from build123d import *

# Parameters (mm, degrees)
BOSS_EXTRUDE6_DEPTH  = 1.27
SKETCH3_R            = 2.54
SKETCH3_R_2          = 1.27
BOSS_EXTRUDE8_DEPTH  = 0.635
BOSS_EXTRUDE10_DEPTH = 5.08
SKETCH4_R            = 1.2065
BOSS_EXTRUDE9_DEPTH  = 1.5748
CHAMFER1_SIZE        = 0.635


with BuildPart() as part:
    # Sketch1 → Boss-Extrude6 (new body)
    with BuildSketch(Plane(origin=(0, 0, 0), x_dir=(1, 0, 0), z_dir=(0, 1, 0))):
        with BuildLine():
            Line((-9.304269575, -27.345620797), (13.511541223, -27.345620797))
            add(Edge.make_bspline(
                [(22.920452389, 30.489026504), (55.478836557, -0.15547818), (13.511541223, -27.345620797)],
                knots=[0, 0, 0, 1, 1, 1], degree=2))
            Line((22.920452389, 30.489026504), (-18.713180741, 30.489026504))
            add(Edge.make_bspline(
                [(-18.713180741, 30.489026504), (-51.271564909, -0.15547818), (-9.304269575, -27.345620797)],
                knots=[0, 0, 0, 1, 1, 1], degree=2))
        make_face()
    extrude(amount=BOSS_EXTRUDE6_DEPTH)

    # Sketch3 → Boss-Extrude8 (add)
    # profile 1 of 8: a face of its own
    with BuildSketch(Plane(origin=(0, 1.27, 0), x_dir=(1, 0, 0), z_dir=(0, 1, 0))):
        with Locations(Location((-15.041364176, 0.374076722, 0), (0, 0, 270))):
            Circle(SKETCH3_R)
        with Locations((-15.041364176, 0.374076722)):
            Circle(SKETCH3_R_2, mode=Mode.SUBTRACT)
    # profile 2 of 8: a face of its own
    with BuildSketch(Plane(origin=(0, 1.27, 0), x_dir=(1, 0, 0), z_dir=(0, 1, 0))):
        with Locations(Location((-3.611364176, 19.48073103, 0), (0, 0, 270))):
            Circle(SKETCH3_R)
        with Locations((-3.611364176, 19.48073103)):
            Circle(SKETCH3_R_2, mode=Mode.SUBTRACT)
    # profile 3 of 8: a face of its own
    with BuildSketch(Plane(origin=(0, 1.27, 0), x_dir=(1, 0, 0), z_dir=(0, 1, 0))):
        with Locations(Location((7.818635824, 19.48073103, 0), (0, 0, 270))):
            Circle(SKETCH3_R)
        with Locations((7.818635824, 19.48073103)):
            Circle(SKETCH3_R_2, mode=Mode.SUBTRACT)
    # profile 4 of 8: a face of its own
    with BuildSketch(Plane(origin=(0, 1.27, 0), x_dir=(1, 0, 0), z_dir=(0, 1, 0))):
        with Locations(Location((19.248635824, 0.374076722, 0), (0, 0, 270))):
            Circle(SKETCH3_R)
        with Locations((19.248635824, 0.374076722)):
            Circle(SKETCH3_R_2, mode=Mode.SUBTRACT)
    # profile 5 of 8: a face of its own
    with BuildSketch(Plane(origin=(0, 1.27, 0), x_dir=(1, 0, 0), z_dir=(0, 1, 0))):
        with Locations((-15.041364176, 0.374076722)):
            Circle(SKETCH3_R_2)
    # profile 6 of 8: a face of its own
    with BuildSketch(Plane(origin=(0, 1.27, 0), x_dir=(1, 0, 0), z_dir=(0, 1, 0))):
        with Locations((-3.611364176, 19.48073103)):
            Circle(SKETCH3_R_2)
    # profile 7 of 8: a face of its own
    with BuildSketch(Plane(origin=(0, 1.27, 0), x_dir=(1, 0, 0), z_dir=(0, 1, 0))):
        with Locations((7.818635824, 19.48073103)):
            Circle(SKETCH3_R_2)
    # profile 8 of 8: a face of its own
    with BuildSketch(Plane(origin=(0, 1.27, 0), x_dir=(1, 0, 0), z_dir=(0, 1, 0))):
        with Locations((19.248635824, 0.374076722)):
            Circle(SKETCH3_R_2)
    extrude(amount=BOSS_EXTRUDE8_DEPTH)

    # Sketch2 → Boss-Extrude10 (add)
    with BuildSketch(Plane(origin=(0, 1.27, 0), x_dir=(1, 0, 0), z_dir=(0, 1, 0))):
        with BuildLine():
            add(Edge.make_bspline(
                [(-32.882940994, 5.946281814), (-32.05929394, 17.927437872), (-18.713180741, 30.489026504)],
                knots=[0.590086746, 0.590086746, 0.590086746, 1, 1, 1], degree=2))
            Line((-32.882940994, 5.946281814), (-30.849557533, 9.46820528))
            add(Edge.make_bspline(
                [(-21.52012223, 25.627261232), (-29.022947824, 17.416183265), (-30.849557533, 9.46820528)],
                knots=[0.061508066, 0.061508066, 0.061508066, 0.343715302, 0.343715302, 0.343715302], degree=2))
            Line((-21.52012223, 25.627261232), (-18.713180741, 30.489026504))
        make_face()
        with BuildLine():
            Line((-30.849557533, 9.46820528), (-32.882940994, 5.946281814))
            Line((-32.882940994, 5.946281814), (-31.432013688, 3.897645158))
            add(Edge.make_bspline(
                [(-31.376148124, 6.016123622), (-31.455454937, 4.954503137), (-31.432013688, 3.897645158)],
                knots=[0.405223368, 0.405223368, 0.405223368, 0.443192049, 0.443192049, 0.443192049], degree=2))
            add(Edge.make_bspline(
                [(-30.849557533, 9.46820528), (-31.247673588, 7.735915333), (-31.376148124, 6.016123622)],
                knots=[0.343715302, 0.343715302, 0.343715302, 0.405223368, 0.405223368, 0.405223368], degree=2))
        make_face()
        with BuildLine():
            add(Edge.make_bspline(
                [(-9.304269575, -27.345620797), (-34.068614317, -11.301078017), (-32.882940994, 5.946281814)],
                knots=[0, 0, 0, 0.590086746, 0.590086746, 0.590086746], degree=2))
            Line((-9.304269575, -27.345620797), (-11.605197436, -24.096825947))
            add(Edge.make_bspline(
                [(-31.432013688, 3.897645158), (-31.111690719, -10.544242355), (-11.605197436, -24.096825947)],
                knots=[0.443192049, 0.443192049, 0.443192049, 0.962031319, 0.962031319, 0.962031319], degree=2))
            Line((-31.432013688, 3.897645158), (-32.882940994, 5.946281814))
        make_face()
        with BuildLine():
            Line((35.056829181, 9.46820528), (37.090212642, 5.946281814))
            add(Edge.make_bspline(
                [(22.920452389, 30.489026504), (36.266565588, 17.927437872), (37.090212642, 5.946281814)],
                knots=[0, 0, 0, 0.409913254, 0.409913254, 0.409913254], degree=2))
            Line((22.920452389, 30.489026504), (25.727393878, 25.627261232))
            add(Edge.make_bspline(
                [(25.727393878, 25.627261232), (33.230219472, 17.416183265), (35.056829181, 9.46820528)],
                knots=[0.061508066, 0.061508066, 0.061508066, 0.343715302, 0.343715302, 0.343715302], degree=2))
        make_face()
        with BuildLine():
            Line((35.639285336, 3.897645158), (37.090212642, 5.946281814))
            Line((37.090212642, 5.946281814), (35.056829181, 9.46820528))
            add(Edge.make_bspline(
                [(35.056829181, 9.46820528), (35.454945236, 7.735915333), (35.583419772, 6.016123622)],
                knots=[0.343715302, 0.343715302, 0.343715302, 0.405223368, 0.405223368, 0.405223368], degree=2))
            add(Edge.make_bspline(
                [(35.583419772, 6.016123622), (35.662726585, 4.954503137), (35.639285336, 3.897645158)],
                knots=[0.405223368, 0.405223368, 0.405223368, 0.443192049, 0.443192049, 0.443192049], degree=2))
        make_face()
        with BuildLine():
            Line((15.812469084, -24.096825947), (13.511541223, -27.345620797))
            add(Edge.make_bspline(
                [(37.090212642, 5.946281814), (38.275885965, -11.301078017), (13.511541223, -27.345620797)],
                knots=[0.409913254, 0.409913254, 0.409913254, 1, 1, 1], degree=2))
            Line((37.090212642, 5.946281814), (35.639285336, 3.897645158))
            add(Edge.make_bspline(
                [(35.639285336, 3.897645158), (35.318962367, -10.544242355), (15.812469084, -24.096825947)],
                knots=[0.443192049, 0.443192049, 0.443192049, 0.962031319, 0.962031319, 0.962031319], degree=2))
        make_face()
        with BuildLine():
            Line((-9.304269575, -27.345620797), (13.511541223, -27.345620797))
            Line((13.511541223, -27.345620797), (15.812469084, -24.096825947))
            add(Edge.make_bspline(
                [(15.812469084, -24.096825947), (14.384983027, -25.088604625), (12.854748908, -26.075620797)],
                knots=[0.962031319, 0.962031319, 0.962031319, 1, 1, 1], degree=2))
            Line((12.854748908, -26.075620797), (-8.64747726, -26.075620797))
            add(Edge.make_bspline(
                [(-11.605197436, -24.096825947), (-10.177711379, -25.088604625), (-8.64747726, -26.075620797)],
                knots=[0.962031319, 0.962031319, 0.962031319, 1, 1, 1], degree=2))
            Line((-11.605197436, -24.096825947), (-9.304269575, -27.345620797))
        make_face()
        with BuildLine():
            Line((25.727393878, 25.627261232), (22.920452389, 30.489026504))
            Line((22.920452389, 30.489026504), (-18.713180741, 30.489026504))
            Line((-18.713180741, 30.489026504), (-21.52012223, 25.627261232))
            add(Edge.make_bspline(
                [(-17.979945899, 29.219026504), (-19.884854823, 27.416894751), (-21.52012223, 25.627261232)],
                knots=[0, 0, 0, 0.061508066, 0.061508066, 0.061508066], degree=2))
            Line((-17.979945899, 29.219026504), (22.187217547, 29.219026504))
            add(Edge.make_bspline(
                [(22.187217547, 29.219026504), (24.092126471, 27.416894751), (25.727393878, 25.627261232)],
                knots=[0, 0, 0, 0.061508066, 0.061508066, 0.061508066], degree=2))
        make_face()
    extrude(amount=BOSS_EXTRUDE10_DEPTH)

    # Sketch4 → Boss-Extrude9 (add)
    with BuildSketch(Plane(origin=(0, 1.905, 0), x_dir=(1, 0, 0), z_dir=(0, 1, 0))):
        with Locations(Location((-15.041364176, 0.374076722, 0), (0, 0, 270))):
            Circle(SKETCH4_R)
        with Locations(Location((-3.611364176, 19.48073103, 0), (0, 0, 270))):
            Circle(SKETCH4_R)
        with Locations(Location((7.818635824, 19.48073103, 0), (0, 0, 270))):
            Circle(SKETCH4_R)
        with Locations(Location((19.248635824, 0.374076722, 0), (0, 0, 270))):
            Circle(SKETCH4_R)
    extrude(amount=BOSS_EXTRUDE9_DEPTH)

    # Chamfer1
    chamfer1_edges = [part.edges().sort_by_distance(p)[0] for p in [
        (2.103635824, 0, 27.345620797),
        (-32.321436727, 0, 0.895081973),
        (36.528708375, 0, 0.895081973),
        (2.103635824, 0, -30.489026504),
    ]]
    chamfer(chamfer1_edges, length=CHAMFER1_SIZE)


solid = part.part
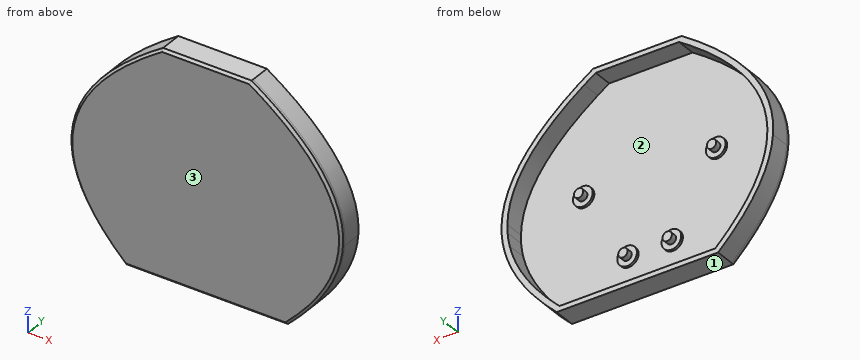
Verification items for the finished model (mm, model axes). Face numbers are marked on the shaded views. Give positions to 0.01 mm unless a question says otherwise; leave off trailing zeros. Loops run counter-clockwise (first coordinate to the right, second up) from the corner with the lowest first, then second, coordinate; pieces in that order, holes last. Notation, with made-up numbers: (-31.75, 88) - (23.25, 88) arc R15 cw to (23.25, 100) - close; hole circle Ø11 at (1, 48). An arc over 180 degrees is marked (long way). Write item = value, one per line. Start each with the question number.
Q1. Cross-section at A-A, the plane x = -7. Enter the section's corners in (y, z) (3 decimals).
Q2. Thickness scan on line 1 (Z direction, x = 10, y = 2); line 2 (X direction, y = 2, z = -5); line 3 (Y direction, x = 11.5, z = 2). Record the ranges inside material, lowest first.
Q3. Depth check by flat-ended pin: P1, Ø1.5, axis at x = -4.5, z = -20.5, coming from the +Y side; P2, Ø4, axis at x = 9.5, z = 10, coming from the +Y side; P3, Ø2, axis at y = 5.5, z = -8, coming from the -X side. Enter the tip coordinate at first touch or a pass-through.
Q4. Mould release check, pull along Z, two halves, no side actions. Record for the marked faces 1, 2 and 3: released by +Z, released by -Z, zero draft, split by the parting line, or undercut.
Answer key:
q1.outline = (0, -29.854) - (0.635, -30.489) - (6.35, -30.489) - (6.35, -29.219) - (1.27, -29.219) - (1.27, 26.076) - (6.35, 26.076) - (6.35, 27.346) - (0.635, 27.346) - (0, 26.711) - close
q2.line_1 = -30.49 to -29.22, 26.08 to 27.35
q2.line_2 = -32.93 to -31.43, 35.64 to 37.14
q2.line_3 = 0 to 1.27
q3.P1 = 3.48
q3.P2 = 1.27
q3.P3 = -32.79
q4.face_1 = released by -Z
q4.face_2 = undercut
q4.face_3 = zero draft
